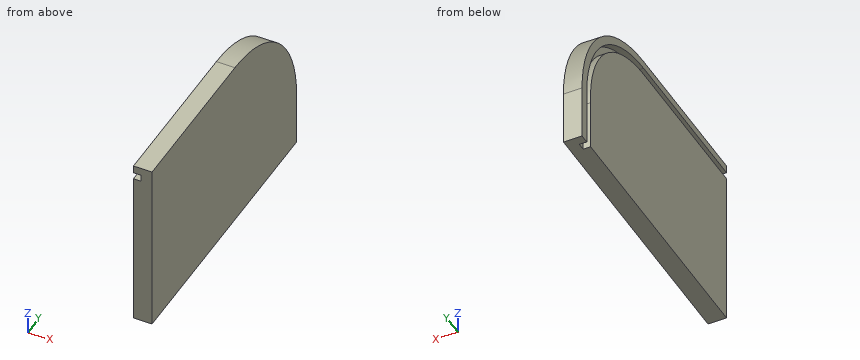
from build123d import *

# Parameters (mm, degrees)
F1_DEPTH = 20
F3_DEPTH = 8


with BuildPart() as f1:
    # F0 (on Right) → F1 (new body)
    with BuildSketch(Plane.YZ):
        with BuildLine():
            Line((0, 76.777947), (-175, 76.777947))
            Line((-175, 76.777947), (-175, -113.118447))
            Line((-175, -113.118447), (129.999959, -113.118447))
            Line((129.999959, -113.118447), (129.999959, -53.118447))
            ThreePointArc((129.999959, -53.118447), (91.887244, 38.738451), (0, 76.777947))
        make_face()
    extrude(amount=F1_DEPTH)

    # F2 (on face) → F3 (cut)
    with BuildSketch(Plane(origin=(0, 0, 0), x_dir=(0, -1, 0), z_dir=(-1, 0, 0))):
        with BuildLine():
            Line((175, 60.811221), (175, 68.414755))
            Line((175, 68.414755), (0, 68.414755))
            ThreePointArc((0, 68.414755), (-87.193236, 30.937351), (-119.999959, -58.118447))
            Line((-119.999959, -58.118447), (-119.999959, -113.118447))
            Line((-119.999959, -113.118447), (-111.999959, -113.118447))
            Line((-111.999959, -113.118447), (-111.999959, -58.118447))
            ThreePointArc((-111.999959, -58.118447), (-81.682704, 25.532649), (0, 60.811221))
            Line((0, 60.811221), (175, 60.811221))
        make_face()
    extrude(amount=-F3_DEPTH, mode=Mode.SUBTRACT)


solid = f1.part
Could you check a few things on this model? Use its own coordinates, in mm. Give positions to 0.01 mm unless a question says otherwise; leave off trailing zeros. Loops run counter-clockwise (first coordinate to the right, second up) from the corner with the lowest first, then second, coordinate; pieces in that order, holes last. Notation, with made-up numbers: M 15,-19.75 L 30,-19.75 A19 cw 30,1.25 Z; hole C 79.5,-36 d11. An arc over 180 degrees is marked long. Answer as a JSON object with one key per item and string values.
Q1. For P1, Ø1.5, axis at x = 16.5, z = -18.5, coming from the +Y side; P2, Ø1.5, axis at y = -65, z = -12.5, coming from the -X side, each with a flat end and sliding along its axis, tell me the tip position at first contact or that it passes through.
Values found:
{"P1": "stops at y = 125.48", "P2": "stops at x = 0"}
Q2. Suppose I cut it at A-A, the plane x = 5. List the corners of the cut face in (y, z) for me.
Values found:
{"outline": "M -175,-113.12 L 112,-113.12 L 112,-58.12 A112.2 ccw 0,60.81 L -175,60.81 Z; M -175,68.41 L 0,68.41 A120.17 cw 120,-58.12 L 120,-113.12 L 130,-113.12 L 130,-53.12 A130 ccw 0,76.78 L -175,76.78 Z"}
Q3. Suppose I cut it at C-C, the plane z = 51.5. List the corners of the cut face in (x, y) for me, plus the area to 3 significant figures.
Values found:
{"outline": "M 0,-175 L 20,-175 L 20,77.03 L 0,77.03 L 0,61.47 L 8,61.47 L 8,44.75 L 0,44.75 Z", "area": "4,910 mm²"}
Q4. Suppose I cut it at B-B, the plane y = -6. List the corners of the cut face in (x, z) for me, plus the area to 3 significant figures.
Values found:
{"outline": "M 0,-113.12 L 20,-113.12 L 20,76.78 L 0,76.78 L 0,68.41 L 8,68.41 L 8,60.81 L 0,60.81 Z", "area": "3,740 mm²"}
Q5. If I drill on probe 1 along Z at (x, y) = (6.75, -162); probe 2 along Y at (x, z) = (5.5, -87.5); probe 3 along Z at (x, y) = (6.25, 48), over which ranges is the centre line in solid material (lowest first)? Write a range as [from, to].
Values found:
{"probe 1": "z = [-113.12, 60.81], [68.41, 76.78]", "probe 2": "y = [-175, 112], [120, 130]", "probe 3": "z = [-113.12, 50.03], [58.41, 67.59]"}
